from build123d import *

# Parameters (mm, degrees)
SKETCH_2_R          = 1.6
CUT_EXTRUDE_1_DEPTH = 10


with BuildPart() as part:
    # 草图1 → 旋转1 (revolve)
    with BuildSketch(Plane.XY, mode=Mode.PRIVATE) as revolve_1_sk:
        Polygon((-9, 0), (-9, 2.45), (-5, 2.45), (-5, 6.25), (0, 6.25), (0, 12), (1.3, 12), (1.3, 6.25), (14.5, 6.25), (14.5, 0), align=None)
    revolve(revolve_1_sk.sketch.rotate(Axis((-8.079555556, 0, 0), (1, 0, 0)), 90), axis=Axis((-8.079555556, 0, 0), (1, 0, 0)))

    # 草图2 → 切除-拉伸1 (cut)
    with BuildSketch(Plane.ZY):
        with Locations((0, 9)):
            Circle(SKETCH_2_R)
        with Locations((7.794228634, -4.5)):
            Circle(SKETCH_2_R)
        with Locations((-7.794228634, -4.5)):
            Circle(SKETCH_2_R)
    extrude(amount=-CUT_EXTRUDE_1_DEPTH, mode=Mode.SUBTRACT)


solid = part.part
Geometry check sheet. Reference: the model listing, model coordinates, mm. A direction names the side the tool comes from. Give positions to 0.01 mm unless a question says otherwise; leave off trailing zeros. Loops run counter-clockwise (first coordinate to the right, second up) from the corner with the lowest first, then second, coordinate; pieces in that order, holes last.
(1) Set-up check for faces 1 (the cylindrical face through (-2.46, -1.88, 5.96)), 2 (the cylindrical face through (0.641, -5.474, -9.064)), 3 (the flat face through (1.3, 5, 5)): record each of +Z, -Z, +X, -X, +Y, -Y from which the full face is reachable in a straight line by a thin tool's end or side.
From the geometry:
face 1: -X
face 2: +X, -X
face 3: +X
(2) Section check D-D on x = -6.25. Record the cut outline in (y, z).
From the geometry:
outline: circle Ø4.9 at (0, 0)
(3) Section check C-C on y = -4.5. Record the cut outline in (x, z), then the cut area to 3 significant figures.
From the geometry:
outline: (-5, -4.34) - (0, -4.34) - (0, -6.19) - (1.3, -6.19) - (1.3, -4.34) - (14.5, -4.34) - (14.5, 4.34) - (1.3, 4.34) - (1.3, 6.19) - (0, 6.19) - (0, 4.34) - (-5, 4.34) - close; (0, -11.12) - (1.3, -11.12) - (1.3, -9.39) - (0, -9.39) - close; (0, 9.39) - (1.3, 9.39) - (1.3, 11.12) - (0, 11.12) - close
area: 178 mm2
(4) Depth check by flat-ended pin: pin 1 Ø2 at (y, z) = (7, 6) entering from -X; pin 2 Ø8 at (x, y) = (2, 4.5) entering from +Z; pin 3 Ø1.5 at (x, y) = (8, -4) entering from +Z. Enter the tip coordinate at first touch or a pass-through.
From the geometry:
pin 1: stops at x = 0
pin 2: stops at z = 11.99
pin 3: stops at z = 5.34
(5) Section check A-A on z = 0. Record the cut outline in (x, y), then the cut area to 3 significant figures.
From the geometry:
outline: (-9, -2.45) - (-5, -2.45) - (-5, -6.25) - (0, -6.25) - (0, -12) - (1.3, -12) - (1.3, -6.25) - (14.5, -6.25) - (14.5, 6.25) - (1.3, 6.25) - (1.3, 7.4) - (0, 7.4) - (0, 6.25) - (-5, 6.25) - (-5, 2.45) - (-9, 2.45) - close; (0, 10.6) - (1.3, 10.6) - (1.3, 12) - (0, 12) - close
area: 274 mm2
(6) Section check B-B on y = 0. Record the cut outline in (x, z).
From the geometry:
outline: (-9, -2.45) - (-5, -2.45) - (-5, -6.25) - (0, -6.25) - (0, -12) - (1.3, -12) - (1.3, -6.25) - (14.5, -6.25) - (14.5, 6.25) - (1.3, 6.25) - (1.3, 12) - (0, 12) - (0, 6.25) - (-5, 6.25) - (-5, 2.45) - (-9, 2.45) - close
(7) Release check for a two-part mould opening along Y. For faces 4 (the flat face through (0, 5, -5)), 5 (the cylindrical face through (0.64, 7.44, -0.35)), 6 (the cylindrical face through (7.99, -1.88, 5.96)) record: released by +Y, released by -Y, zero draft, split by the parting line, or undercut.
From the geometry:
face 4: zero draft
face 5: undercut
face 6: split by the parting line
(8) Thickness scan on L1, parallel to X at y = 4.25, z = -6; L2, parallel to Y at x = 0.55, z = 0; L3, parallel to X at y = 4.5, z = 1.5. Record the ranges inside material, lowest first.
From the geometry:
L1: x = 0 to 1.3
L2: y = -12 to 7.4, 10.6 to 12
L3: x = -5 to 14.5
